Verification items for the finished model (mm, model axes). A direction names the side the tool comes from. Give positions to 0.01 mm unless a question says otherwise; leave off trailing zeros. Loops run counter-clockwise (first coordinate to the right, second up) from the corner with the lowest first, then second, coordinate; pieces in that order, holes last. Notation, with made-up numbers: M 3.25,37.25 L 43.25,37.25 A26 cw 43.25,57.25 Z; hole C 70.25,-19.5 d6. An arc over 180 degrees is marked long. Answer in a Markdown table with one row per item.
Autodesk Fusion 360 part; units mm, degrees
sketch "スケッチ1" plane through (0, 0, 0) normal (0, 1, 0) x (1, 0, 0)
  line L0 (25.25, -27) -> (-25.25, -27)
  line L1 (-25.25, -27) -> (-25.25, 27)
  line L2 (-25.25, 27) -> (25.25, 27)
  line L3 (25.25, 27) -> (25.25, -27)
  line L4 (25.25, -27) -> (-25.25, 27) construction
  line L5 (-25.25, -27) -> (25.25, 27) construction
  dimension "d1" = 50.5
  dimension "d2" = 54
sketch "スケッチ2" plane through (12.875, 0, 0) normal (1, 0, 0) x (0, 0, -1)
  line L0 (-25, 2) -> (25, 2)
  line L1 (25, 2) -> (25, 12)
  line L2 (25, 12) -> (-25, 12)
  line L3 (-25, 12) -> (-25, 2)
  line L4 (25, 2) -> (7, 2) construction
  line L5 (7, 2) -> (7, 4) construction
  line L6 (7, 4) -> (25, 4) construction
  line L7 (25, 4) -> (25, 2) construction
  line L8 (7, 4) -> (-7, 4)
  line L9 (-7, 4) -> (-7, 12)
  line L10 (-7, 12) -> (7, 12)
  line L11 (7, 12) -> (7, 4)
  dimension "d7" = 18
  dimension "d8" = 2
  dimension "d11" = 14
sketch "スケッチ3" plane through (0, 2, 0) normal (0, 1, 0) x (-1, 0, 0)
  circle A0 centre (-6.1875, 18.4923) radius 1.75
  line L0 (-0.5, -25) -> (-0.5, 25)
  line L1 (-0.5, 25) -> (-11.875, 25)
  line L2 (-11.875, 25) -> (-11.875, -25)
  line L3 (-11.875, -25) -> (-0.5, -25)
  line L4 (-6.1875, 18.4923) -> (6.1875, 18.4923) construction
  line L5 (6.1875, 18.4923) -> (6.1875, -18.4923) construction
  line L6 (6.1875, -18.4923) -> (-6.1875, -18.4923) construction
  line L7 (-6.1875, -18.4923) -> (-6.1875, 18.4923) construction
  circle A1 centre (6.1875, -18.4923) radius 1.75
  dimension "d12" = 12.375
  dimension "d13" = 36.9846
  dimension "d14" = 3.5
sketch "スケッチ4" plane through (0, 2, 0) normal (0, 1, 0) x (-1, 0, 0)
  line L0 (-0.5, -25) -> (-0.5, 25)
  line L1 (-0.5, 25) -> (-11.875, 25)
  line L2 (-11.875, 25) -> (-11.875, -25)
  line L3 (-11.875, -25) -> (-0.5, -25)
  line L4 (-11.875, 25) -> (-6.1875, 25) construction
  line L5 (-6.1875, 25) -> (-6.1875, 18.4923) construction
  line L6 (-6.1875, 18.4923) -> (-11.875, 18.4923) construction
  line L7 (-11.875, 18.4923) -> (-11.875, 25) construction
  circle A0 centre (-6.1875, 18.4923) radius 1.75
  dimension "d17" = 5.6875
  dimension "d18" = 6.5077
  dimension "d19" = 3.5
sketch "スケッチ5" plane through (0, 2, 0) normal (0, 1, 0) x (-1, 0, 0)
  line L0 (0.5, 25) -> (0.5, -25)
  line L1 (0.5, -25) -> (24.25, -25)
  line L2 (24.25, -25) -> (24.25, 25)
  line L3 (24.25, 25) -> (0.5, 25)
  line L4 (0.5, -25) -> (11.875, -25) construction
  line L5 (11.875, -25) -> (11.875, 25) construction
  line L6 (11.875, 25) -> (0.5, 25) construction
  line L7 (0.5, 25) -> (0.5, -25) construction
  line L8 (11.875, -25) -> (12.875, -25)
  line L9 (12.875, -25) -> (12.875, 25)
  line L10 (12.875, 25) -> (11.875, 25)
  line L11 (11.875, 25) -> (11.875, -25)
  dimension "d20" = 50
  dimension "d23" = 11.375
  dimension "d24" = 1
  dimension "d25" = 50
sketch "スケッチ6" plane through (0, 2, 0) normal (0, 1, 0) x (-1, 0, 0)
  line L0 (-11.875, 25) -> (-11.875, -25)
  line L1 (-11.875, -25) -> (24.25, -25)
  line L2 (24.25, -25) -> (24.25, 25)
  line L3 (24.25, 25) -> (-11.875, 25)
  line L4 (-11.875, -25) -> (-0.5, -25) construction
  line L5 (-0.5, -25) -> (-0.5, 25) construction
  line L6 (-0.5, 25) -> (-11.875, 25) construction
  line L7 (-11.875, 25) -> (-11.875, -25) construction
  line L8 (-0.5, -25) -> (0.5, -25)
  line L9 (0.5, -25) -> (0.5, 25)
  line L10 (0.5, 25) -> (-0.5, 25)
  line L11 (-0.5, 25) -> (-0.5, -25)
  dimension "d26" = 11.375
  dimension "d29" = 50
  dimension "d30" = 50
  dimension "d31" = 1
sketch "スケッチ7" plane through (0, 2, 0) normal (0, 1, 0) x (-1, 0, 0)
  line L0 (-24.25, -25) -> (24.25, -25)
  line L1 (24.25, -25) -> (24.25, 25)
  line L2 (24.25, 25) -> (-24.25, 25)
  line L3 (-24.25, 25) -> (-24.25, -25)
  line L4 (-24.25, -25) -> (-12.875, -25) construction
  line L5 (-12.875, -25) -> (-12.875, 25) construction
  line L6 (-12.875, 25) -> (-24.25, 25) construction
  line L7 (-24.25, 25) -> (-24.25, -25) construction
  line L8 (-12.875, -25) -> (-11.875, -25)
  line L9 (-11.875, -25) -> (-11.875, 25)
  line L10 (-11.875, 25) -> (-12.875, 25)
  line L11 (-12.875, 25) -> (-12.875, -25)
  dimension "d38" = 50
  dimension "d39" = 11.375
  dimension "d40" = 50
  dimension "d43" = 1
sketch "スケッチ8" plane through (12.875, 0, 0) normal (1, 0, 0) x (0, 0, -1)
  line L0 (7, 12) -> (7, 4)
  line L1 (7, 4) -> (-7, 4)
  line L2 (-7, 4) -> (-7, 12)
  line L3 (-7, 12) -> (-25, 12)
  line L4 (-25, 12) -> (-25, 2)
  line L5 (-25, 2) -> (25, 2)
  line L6 (25, 2) -> (25, 12)
  line L7 (25, 12) -> (7, 12)
  line L8 (7, 4) -> (25, 12)
  line L9 (25, 12) -> (7, 12)
  line L10 (7, 12) -> (7, 4)
sketch "スケッチ9" plane through (12.875, 0, 0) normal (1, 0, 0) x (0, 0, -1)
  line L0 (25, 12) -> (7, 4)
  line L1 (7, 4) -> (-7, 4)
  line L2 (-7, 4) -> (-7, 12)
  line L3 (-7, 12) -> (-25, 12)
  line L4 (-25, 12) -> (-25, 2)
  line L5 (-25, 2) -> (25, 2)
  line L6 (25, 2) -> (25, 12)
  line L7 (-7, 12) -> (-7, 4)
  line L8 (-7, 12) -> (-25, 12)
  line L9 (-7, 4) -> (-25, 12)
sketch "スケッチ10" plane through (0, 13, 0) normal (0, 1, 0) x (-1, 0, 0)
  line L0 (20.25, -27) -> (20.25, 27)
  line L1 (20.25, 27) -> (-20.25, 27)
  line L2 (-20.25, 27) -> (-20.25, -27)
  line L3 (-20.25, -27) -> (20.25, -27)
  line L4 (-24.25, 25) -> (24.25, 25)
  line L5 (24.25, 25) -> (24.25, -25)
  line L6 (24.25, -25) -> (-24.25, -25)
  line L7 (-24.25, -25) -> (-24.25, 25)
  line L8 (-24.25, 25) -> (24.25, -25) construction
  line L9 (24.25, 25) -> (-24.25, -25) construction
  dimension "d44" = 48.5
  dimension "d45" = 50
extrude "押し出し1" add sketch "スケッチ1" along normal blind 13
fillet "フィレット1" radius 5 1 edges at (25.25, 13, 0)
fillet "フィレット2" radius 5 1 edges at (-25.25, 13, 0)
extrude "押し出し2" cut sketch "スケッチ10" against normal blind 11 contours L0 L2 L4 L6 | L0 L4 L5 L6 | L2 L4 L6 L7
extrude "押し出し3" add sketch "スケッチ7" along normal blind 10 contours L0 L2 L8 L9 L10 L11
extrude "押し出し4" add sketch "スケッチ6" along normal blind 10 contours L1 L3 L8 L9 L10 L11
extrude "押し出し5" add sketch "スケッチ5" along normal blind 10 contours L1 L3 L8 L9 L10 L11
extrude "押し出し6" cut sketch "スケッチ2" against normal blind 28 contours L2 L8 L9 L10 L11
extrude "押し出し7" cut sketch "スケッチ8" against normal blind 27 contours L0 L7 L8 L9 L10
extrude "押し出し8" cut sketch "スケッチ9" against normal blind 28 contours L2 L3 L7 L8 L9
extrude "押し出し9" cut sketch "スケッチ4" against normal blind 12 contours A0
extrude "押し出し10" cut sketch "スケッチ3" against normal blind 2 contours A1
Item 1: Release check for a two-part mould opening along X. For faces 3 (the flat face through (6, 2, 0)), 4 (the flat face through (0, 6, -27)), 5 (the cylindrical face through (25.094, 9.241, 0.378)), 6 (the flat face through (-6, 2, 0)) record: released by +X, released by -X, zero draft, split by the parting line, or undercut.
Reported:
| item | result |
|---|---|
| face 3 | undercut |
| face 4 | zero draft |
| face 5 | released by +X |
| face 6 | undercut |
Item 2: Sectioned sample at D-D (x = 5.5). Record the cut outline in (y, z).
Reported:
| item | result |
|---|---|
| outline | M 0,-27 L 13,-27 L 13,-25 L 2,-25 L 2,16.88 L 0,16.88 Z; M 0,20.1 L 2,20.1 L 2,25 L 13,25 L 13,27 L 0,27 Z |
Item 3: Go/stop test with flat-tipped pins: pin 1 (0.5 mm diameter, centred on x = 12.5, z = -3, fed in from +Y); pin 2 (12 mm diameter, centred on x = 5, z = -2, fed in from -Y); pin 3 (4 mm diameter, centred on x = 6.19, z = 18.49, fed in from +Y); pin 4 (1.5 mm diameter, centred on y = 9.5, z = -11, fed in from +X). Record where each tip stops, or that it passes through.
Reported:
| item | result |
|---|---|
| pin 1 | stops at y = 4 |
| pin 2 | stops at y = 0 |
| pin 3 | stops at y = 2 |
| pin 4 | stops at x = 25.19 |
Item 4: Scan lines: L1, parallel to X at y = 2.75, z = -11 (3 decimals); L2, parallel to Z at x = 11, y = 10.25; L3, parallel to X at y = 7, z = 0.5. Record each from-to range of solid material in increasing order. Write a range as [from, to].
Reported:
| item | result |
|---|---|
| L1 | x = [-25.25, -24.25], [-12.875, -11.875], [-0.5, 0.5], [11.875, 12.875], [24.25, 25.25] |
| L2 | z = [-27, -25], [25, 27] |
| L3 | x = [-25.25, -24.25], [24.25, 25.25] |
Item 5: Tool access check on faces 1 (the cylindrical face through (-5.8, 1, -20.2)), 2 (the flat face through (19, 2, 0)). Record the directions out of +Z, -Z, +X, -X, +Y, -Y that give a thin tool (end or side, any length) a straight path to the whole face; none if there is none.
Reported:
| item | result |
|---|---|
| face 1 | +Y, -Y |
| face 2 | +Y |
Item 6: Sectioned sample at C-C (z = 11.5). Record the cut outline in (x, y) (3 decimals).
Reported:
| item | result |
|---|---|
| outline | M -25.25,0 L 25.25,0 L 25.25,8 A5 ccw 24.25,11 L 24.25,2 L 12.875,2 L 12.875,6 L 11.875,6 L 11.875,2 L 0.5,2 L 0.5,6 L -0.5,6 L -0.5,2 L -11.875,2 L -11.875,6 L -12.875,6 L -12.875,2 L -24.25,2 L -24.25,11 A5 ccw -25.25,8 Z |
Item 7: Sectioned sample at A-A (x = -3). Record the cut outline in (y, z), and give its area (3 significant figures).
Reported:
| item | result |
|---|---|
| outline | M 0,-27 L 13,-27 L 13,-25 L 2,-25 L 2,25 L 13,25 L 13,27 L 0,27 Z |
| area | 152 mm^2 |
